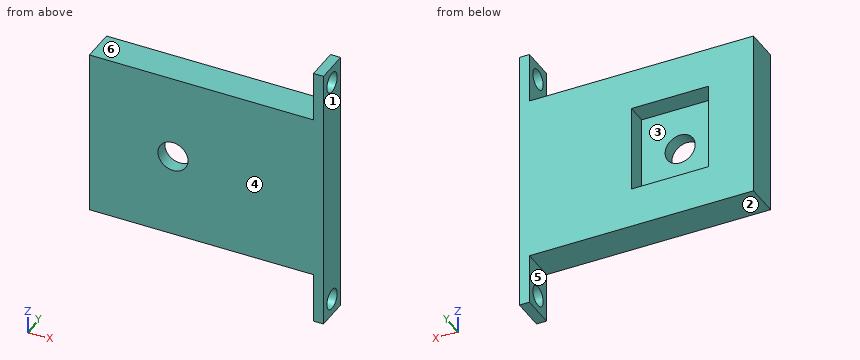
Autodesk Inventor part; units mm, degrees
ref_plane "YZ Plane" through (0, 0, 0) normal (1, 0, 0) x (0, 1, 0)
ref_plane "XZ Plane" through (0, 0, 0) normal (0, 1, 0) x (-1, 0, 0)
ref_plane "XY Plane" through (0, 0, 0) normal (0, 0, 1) x (1, 0, 0)
sketch "Эскиз1" plane through (0, 0, 0) normal (0, 1, 0) x (-1, 0, 0)
  line L0 (0, 0) -> (-70, 0)
  line L1 (-70, 0) -> (-70, -50)
  line L2 (-70, -50) -> (0, -50)
  line L3 (0, -50) -> (0, 0)
  line L4 (-70, 0) -> (-25, 0)
  line L5 (-25, 0) -> (-25, -25)
  line L6 (-25, -25) -> (-70, -25)
  line L7 (-70, -25) -> (-70, 0)
  circle A0 centre (-25, -25) radius 4.5
  line L8 (-70, -50) -> (-70, -65)
  line L9 (-70, -65) -> (-67, -65)
  line L10 (-67, -65) -> (-67, -50)
  line L11 (-70, 0) -> (-70, 15)
  line L12 (-70, 15) -> (-67, 15)
  line L13 (-67, 15) -> (-67, 0)
  point P0 (-67, 0)
  dimension "d0" = 70
  dimension "d1" = 50
  dimension "d2" = 45
  dimension "d3" = 25
  dimension "d4" = 9
  dimension "d31" = 15
  dimension "d32" = 3
  dimension "d33" = 15
  dimension "d34" = 3
extrude "Выдавливание1" add sketch "Эскиз1" along normal blind 4 contours L3 L2 L1 L6 A0 L5 L0 | L5 A0 L6 L1 L0 | L0 L11 L12 L13 | L10 L9 L8 L2
sketch "Эскиз2" plane through (0, 4, 0) normal (0, 1, 0) x (1, 0, 0)
  circle A0 centre (25, 25) radius 4.5
  line L0 (25, 25) -> (25, 12)
  line L1 (25, 12) -> (13.5, 12)
  line L2 (13.5, 12) -> (36.5, 12)
  line L3 (36.5, 12) -> (36.5, 38)
  line L4 (36.5, 38) -> (13.5, 38)
  line L5 (13.5, 38) -> (13.5, 12)
  line L6 (67, 50) -> (0, 50)
  line L7 (0, 0) -> (70, 0)
  line L8 (70, 0) -> (70, 50)
  line L9 (70, 50) -> (0, 50)
  line L10 (0, 50) -> (0, 0)
  line L11 (70, -15) -> (70, 65)
  line L12 (67, 65) -> (67, 50)
  line L13 (70, 65) -> (67, 65)
  line L14 (67, 65) -> (67, 50)
  line L15 (67, 50) -> (70, 50)
  line L16 (70, 50) -> (70, 65)
  line L17 (67, -15) -> (70, -15)
  line L18 (67, 0) -> (67, -15)
  line L19 (70, -15) -> (67, -15)
  line L20 (67, -15) -> (67, 0)
  line L21 (67, 0) -> (70, 0)
  line L22 (70, 0) -> (70, -15)
  dimension "d7" = 13
  dimension "d8" = 11.5
  dimension "d9" = 23
  dimension "d10" = 26
extrude "Выдавливание2" add sketch "Эскиз2" along normal blind 6 contours L9 L8 L7 L10 L6 | L12 L13 L11 L9 | L11 L17 L18 L7
sketch "Эскиз4" plane through (70, 0, 15) normal (1, 0, 0) x (0, 0, -1)
  line L0 (0, 0) -> (0, 10)
  line L1 (0, 5) -> (5, 5)
  line L2 (80, 0) -> (80, 10)
  line L3 (80, 5) -> (75, 5)
  circle A0 centre (5, 5) radius 3
  circle A1 centre (75, 5) radius 3
  point P0 (15, 0)
  dimension "d35" = 5
  dimension "d36" = 5
  dimension "d37" = 6
  dimension "d38" = 6
extrude "Выдавливание4" cut sketch "Эскиз4" against normal blind 3.75
properties part number "Стенка энкодер"
Model file for the job. Use its own axes, mm. Face numbers are marked on the shaded views. A direction names the side the tool comes from. Coordinates: 2 decimals unless noted, no trailing zeros. Loops run counter-clockwise (first coordinate to the right, second up) from the corner with the lowest first, then second, coordinate; pieces in that order, holes last. Notation, with made-up numbers: (55.5, 9.5) - (67.5, 9.5) arc R18 cw to (67.5, 16.5) - close; hole circle Ø8 at (-31.75, 76.5). An arc over 180 degrees is marked (long way). Write item = value, one per line. Start each with the question number.
Item 1: Drop flat-ended pins along their axis: pin 1 Ø1.8 at (x, y) = (23.5, 6) entering from -Z; pin 2 Ø11.5 at (x, z) = (22.5, -25) entering from +Y; pin 3 Ø5 at (x, y) = (27.5, 5.5) entering from +Z. Give the stop position or say it passes through.
Item 2: Saw through at A-A, the plane z = -25. List the corners of the cut face in (x, y), then the cut area to 3 significant figures.
Item 3: Saw through at B-B, the plane x = 25. List the corners of the cut face in (y, z), then the cut area to 3 significant figures.
Item 4: Saw through at C-C, the plane y = 5. List the corners of the cut face in (x, z), then the cut area to 3 significant figures.
Item 5: Pull direction Z, two halves, no side cores. Call the marked faces 1, 2 and 3: +Z half, -Z half, draft (parallel to the pull), parting line (faces both ways), or undercut.
Item 6: 3-axis set-ups, long thin cutter, end or side, ignore diameter. For the marked faces 4, 5 and 6: which of +Z, -Z, +X, -X, +Y, -Y reach the whole face in a straight line?
Item 7: Saw through at D-D, the plane z = -60. List the corners of the cut face in (x, y), then the cut area to 3 significant figures.
Item 8: Wall check: probe 1 along Y at (x, z) = (68, 10); probe 2 along Z at (x, y) = (16, 8); probe 3 along X at (y, z) = (6.25, -24.5). Give the ranges that are in metal, low to high. Write a range as [from, to].
Answers:
q1.pin_1 = -50
q1.pin_2 = 4
q1.pin_3 = 0
q2.outline = (0, 0) - (20.5, 0) - (20.5, 4) - (13.5, 4) - (13.5, 10) - (0, 10) - close; (29.5, 0) - (70, 0) - (70, 10) - (36.5, 10) - (36.5, 4) - (29.5, 4) - close
q2.area = 526 mm2
q3.outline = (0, -50) - (10, -50) - (10, -38) - (4, -38) - (4, -29.5) - (0, -29.5) - close; (0, -20.5) - (4, -20.5) - (4, -12) - (10, -12) - (10, 0) - (0, 0) - close
q3.area = 308 mm2
q4.outline = (0, -50) - (67, -50) - (67, -57) - (70, -57) - (70, 7) - (67, 7) - (67, 0) - (0, 0) - close; (67, -65) - (70, -65) - (70, -63) - (67, -63) - close; (67, 13) - (70, 13) - (70, 15) - (67, 15) - close; hole (13.5, -38) - (36.5, -38) - (36.5, -12) - (13.5, -12) - close
q4.area = 2,960 mm2
q5.face_1 = draft
q5.face_2 = -Z half
q5.face_3 = undercut
q6.face_4 = +Z, -Z, +X, -X, -Y
q6.face_5 = -Z, -X, +Y, -Y
q6.face_6 = +Z, -X, +Y, -Y
q7.outline = (67, 0) - (70, 0) - (70, 2) - (67, 2) - close; (67, 8) - (70, 8) - (70, 10) - (67, 10) - close
q7.area = 12.0 mm2
q8.probe_1 = [0, 2], [8, 10]
q8.probe_2 = [-50, -38], [-12, 0]
q8.probe_3 = [0, 13.5], [36.5, 70]
